The listing builds one solid part. Answer for the finished solid, in the listing's coordinates (mm). A direction names the side the tool comes from. Give positions to 0.01 mm unless a question says otherwise; leave off trailing zeros. Loops run counter-clockwise (first coordinate to the right, second up) from the corner with the lowest first, then second, coordinate; pieces in that order, holes last. Notation, with made-up numbers: M 11.5,28.25 L 17.5,28.25 A18 ccw 17.5,38.25 Z; hole C 44,81 d6. An arc over 180 degrees is marked long. Return JSON: item names as keys, results as strings.
from build123d import *

# Parameters (mm, degrees)
SKIZZE1_W                       = 15
SKIZZE1_H                       = 3.7
SKIZZE1_H_2                     = 3.6
SKIZZE1_H_3                     = 3.5
SKIZZE1_H_4                     = 3.4
AUFSATZ_LINEAR_AUSTRAGEN1_DEPTH = 4


with BuildPart() as part:
    # Skizze1 → Aufsatz-Linear austragen1 (new body)
    with BuildSketch(Plane.XY):
        Polygon((5.9, 35), (5.9, 31), (20.6, 31), (20.6, 35), (30.6, 35), (30.6, 31), (45.2, 31), (45.2, 35), (55.2, 35), (55.2, 31), (69.7, 31), (69.7, 35), (79.7, 35), (79.7, 31), (94.1, 31), (94.1, 35), (100, 35), (100, 0), (0, 0), (0, 23), (5, 23), (5, 24), (0, 24), (0, 35), align=None)
        with Locations((13.4, 11.85)):
            Rectangle(SKIZZE1_W, SKIZZE1_H, mode=Mode.SUBTRACT)
        with Locations((38.4, 11.8)):
            Rectangle(SKIZZE1_W, SKIZZE1_H_2, mode=Mode.SUBTRACT)
        with Locations((62.7, 11.75)):
            Rectangle(SKIZZE1_W, SKIZZE1_H_3, mode=Mode.SUBTRACT)
        with Locations((87.2, 11.7)):
            Rectangle(SKIZZE1_W, SKIZZE1_H_4, mode=Mode.SUBTRACT)
    extrude(amount=AUFSATZ_LINEAR_AUSTRAGEN1_DEPTH)


solid = part.part
(1) A tool of negligible diameter and unlimited length cuts with its end or side. For faces 4 (the flat face through (5.9, 33, 2)), 5 (the flat face through (3, 35, 2)), 6 (the flat face through (30.9, 12, 2)), from which of +Z, -Z, +X, -X, +Y, -Y can it reach the whole face along a straight path? Write none if from no direction.
Values follow:
{"face 4": "+Z, -Z, +Y", "face 5": "+Z, -Z, +X, -X, +Y", "face 6": "+Z, -Z"}
(2) The part is cut by section D-D (z = 3.2). Give the number of separate pieces and of enclosed holes in the cut face, and give its area (3 significant figures).
Values follow:
{"separate pieces": "1", "enclosed holes": "4", "area": "3,050 mm²"}
(3) Given pin 1 (1.2 mm diameter, centred on x = 12, z = 2, fed in from +Y); pin 2 (2 mm diameter, centred on y = 33, z = 2.5, fed in from -X), each flat-ended and moving along its own axis, determine where each tip first touches the part or whether it passes through.
Values follow:
{"pin 1": "y = 31", "pin 2": "x = 0"}
(4) The part is cut by section C-C (x = 66). Determine the outline of the cut face in (y, z).
Values follow:
{"outline": "M 0,0 L 10,0 L 10,4 L 0,4 Z; M 13.5,0 L 31,0 L 31,4 L 13.5,4 Z"}
(5) The part is cut by section A-A (x = 17). Determine the outline of the cut face in (y, z), and give its area (3 significant figures).
Values follow:
{"outline": "M 0,0 L 10,0 L 10,4 L 0,4 Z; M 13.7,0 L 31,0 L 31,4 L 13.7,4 Z", "area": "109 mm²"}
(6) Straight lines are drawn through the part: line 1 along X through (y, z) = (11.5, 2.4); line 2 along Y through (x, z) = (94, 0.25); line 3 along Y through (x, z) = (31.5, 3.15). For each, find the intervals that lie inside material, in ascending order.
Values follow:
{"line 1": "0 to 5.9, 20.9 to 30.9, 45.9 to 55.2, 70.2 to 79.7, 94.7 to 100", "line 2": "0 to 10, 13.4 to 31", "line 3": "0 to 10, 13.6 to 31"}
(7) Determine the mould class of faces 1 (the flat face through (79.7, 33, 2)), 2 (the flat face through (100, 18, 2)), 3 (the flat face through (75, 35, 2)) for opening direction X: released by +X, released by -X, zero draft, split by the parting line, or undercut.
Values follow:
{"face 1": "undercut", "face 2": "released by +X", "face 3": "zero draft"}
(8) The part is cut by section B-B (y = 11). Determine the outline of the cut face in (x, z).
Values follow:
{"outline": "M 0,0 L 5.9,0 L 5.9,4 L 0,4 Z; M 20.9,0 L 30.9,0 L 30.9,4 L 20.9,4 Z; M 45.9,0 L 55.2,0 L 55.2,4 L 45.9,4 Z; M 70.2,0 L 79.7,0 L 79.7,4 L 70.2,4 Z; M 94.7,0 L 100,0 L 100,4 L 94.7,4 Z"}
